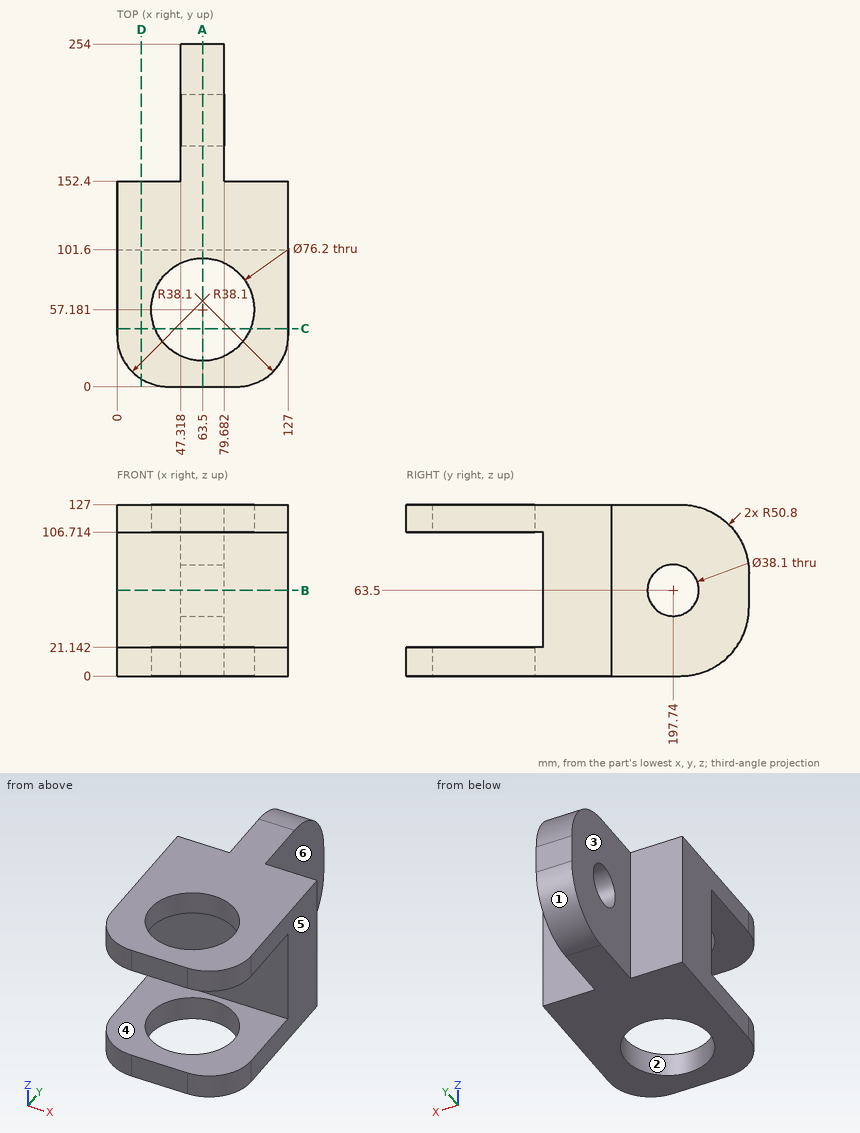
The figure shows three views and two pictorial views of one solid part (mm, origin at its lowest corner). Answer the questions. A direction names the side the tool comes from. Round coordinates to 2 decimals unless told otherwise and drop trailing zeros. Write each loop counter-clockwise with the first axis right and the second up, starting at its lowest first coordinate (ties: lowest second). Pieces come first, ordered by that corner, then holes. Notation, with made-up numbers: (43, 46.5) - (87, 46.5) arc R15 ccw to (87, 51.5) - close; hole circle Ø8 at (34.25, 1.25). An arc over 180 degrees is marked (long way). Answer in a Markdown table with one row per item. Add a question column.
1. A cutting plane is placed at A-A, the plane x = 63.5. Determine the outline of the cut face in (y, z).
2. For the marked faces 4, 5 and 6, determine the directions among +Z, -Z, +X, -X, +Y, -Y from which every point of the face is accessible in a straight line to the end or side of a thin tool.
3. A cutting plane is placed at C-C, the plane y = 43. Determine the outline of the cut face in (x, z).
4. The mould has two halves that part along X. Classify the marked faces 1, 2 and 3: +X half, -X half, draft (parallel to the pull), parting line (faces both ways), or undercut.
5. A cutting plane is placed at D-D, the plane x = 18. Determine the outline of the cut face in (y, z), and give its area (3 significant figures).
6. A cutting plane is placed at B-B, the plane z = 63.5. Determine the outline of the cut face in (x, y).
7. Given pin 1 (14 mm diameter, centred on x = 28, z = 87, fed in from +Y); pin 2 (23 mm diameter, centred on y = 197.74, z = 63.5, fed in from -X); pin 3 (6 mm diameter, centred on y = 210.5, z = 36.5, fed in from +X); pin 4 (4 mm diameter, centred on y = 170, z = 49.5, fed in from -X), each flat-ended and moving along its own axis, determine where each tip first touches the part or whether it passes through.
8. Find the intervals of material crossed by line 1 along Z through (x, y) = (115, 66); line 2 along X through (y, z) = (184.5, 107.5); line 3 along Y through (x, z) = (101, 48), in increasing order. Write a range as from..to.
Worked out:
| question | item | result |
|---|---|---|
| 1 | outline | (0, 0) - (19.08, 0) - (19.08, 21.14) - (0, 21.14) - close; (0, 106.71) - (19.08, 106.71) - (19.08, 127) - (0, 127) - close; (95.28, 0) - (203.2, 0) arc R50.8 ccw to (254, 50.8) - (254, 76.2) arc R50.8 ccw to (203.2, 127) - (95.28, 127) - (95.28, 106.71) - (101.6, 106.71) - (101.6, 21.14) - (95.28, 21.14) - close; hole circle Ø38.1 at (197.74, 63.5) |
| 2 | face 4 | +X, -X, -Y |
| 2 | face 5 | +Z, -Z, +X, +Y, -Y |
| 2 | face 6 | +Z, -Z, +X, +Y |
| 3 | outline | (0, 0) - (28.14, 0) - (28.14, 21.14) - (0, 21.14) - close; (0, 106.71) - (28.14, 106.71) - (28.14, 127) - (0, 127) - close; (98.86, 0) - (127, 0) - (127, 21.14) - (98.86, 21.14) - close; (98.86, 106.71) - (127, 106.71) - (127, 127) - (98.86, 127) - close |
| 4 | face 1 | draft |
| 4 | face 2 | undercut |
| 4 | face 3 | -X half |
| 5 | outline | (5.73, 0) - (152.4, 0) - (152.4, 127) - (5.73, 127) - (5.73, 106.71) - (101.6, 106.71) - (101.6, 21.14) - (5.73, 21.14) - close |
| 5 | area | 10,400 mm^2 |
| 6 | outline | (0, 101.6) - (127, 101.6) - (127, 152.4) - (79.68, 152.4) - (79.68, 178.69) - (47.32, 178.69) - (47.32, 152.4) - (0, 152.4) - close; (47.32, 216.79) - (79.68, 216.79) - (79.68, 254) - (47.32, 254) - close |
| 7 | pin 1 | y = 152.4 |
| 7 | pin 2 | through |
| 7 | pin 3 | x = 79.68 |
| 7 | pin 4 | x = 47.32 |
| 8 | line 1 | 0..21.14, 106.71..127 |
| 8 | line 2 | 47.32..79.68 |
| 8 | line 3 | 101.6..152.4 |
